Geometry check sheet. Reference: the model listing, model coordinates, mm. A direction names the side the tool comes from. Round coordinates to 2 decimals unless told otherwise and drop trailing zeros. Write each loop counter-clockwise with the first axis right and the second up, starting at its lowest first coordinate (ties: lowest second). Pieces come first, ordered by that corner, then holes.
Item 1: Cross-section at A-A (z = -9). Enter the section's corners in (x, y) (3 decimals), then the cut area to 3 significant figures.
Item 2: Scan lines: probe 1 along X at (y, z) = (0, -8.5); probe 2 along Y at (x, z) = (-0.5, -11.25); probe 3 along Y at (x, z) = (1, -2.75). Record each from-to range of solid material in increasing order.
Item 3: Draft check along X on faces 3 (the face through (-3.3, -5.6, -3.2)), 4 (the face through (0, 0, -13)), 5 (the face through (3.32, 0.74, -5.6)), 6 (the face through (3.3, 5.6, -3.2)). Enter one of: pulls with the +X half, pulls with the -X half, needs draft (parallel to the pull), parting line crosses it, or undercut.
Item 4: Access from +Z, -Z, +X, -X, +Y, -Y to the whole of each face (thin tool, end or side, straight path). Record for faces 1 (the face through (1.3, -4.1, 0)), 2 (the face through (1.88, 5.96, -7.61)).
Item 5: Depth check by flat-ended pin: P1, Ø4, axis at x = 0, y = 0, coming from the +Z side; P2, Ø1.5, axis at x = -4.5, y = 2.5, coming from the -Z side; P3, Ø1.5, axis at x = -4, y = -3, coming from the +Z side; P4, Ø8, axis at y = -4, z = -10.5, coming from the +X side. Enter the tip coordinate at first touch or a pass-through.
Item 6: Cross-section at B-B (z = -14). Enter the section's corners in (x, y), then the cut area to 3 significant figures.
from build123d import *

# Parameters (mm, degrees)
BOSS_EXTRUDE1_DEPTH = 15


with BuildPart() as part:
    # Sketch1 → Boss-Extrude1 (new body)
    with BuildSketch(Plane.XY):
        Polygon((0, 7.505553499), (-6.5, 3.75277675), (-6.5, -3.75277675), (0, -7.505553499), (6.5, -3.75277675), (6.5, 3.75277675), align=None)
    extrude(amount=-BOSS_EXTRUDE1_DEPTH)

    # Sketch2 → Cut-Revolve7 (revolve, cut)
    with BuildSketch(Plane(origin=(0, 0, 0), x_dir=(0, 0, -1), z_dir=(1, 0, 0))):
        with BuildLine():
            Line((16, 0), (15, 0))
            ThreePointArc((15, 0), (13.169417382, 4.419417382), (8.75, 6.25))
            Line((8.75, 6.25), (6.5, 6.25))
            Line((6.5, 6.25), (6.5, 30.553605498))
            Line((6.5, 30.553605498), (16, 30.553605498))
            Line((16, 30.553605498), (16, 0))
        make_face()
    revolve(axis=Axis((0, 0, 0), (0, 0, -1)), mode=Mode.SUBTRACT)

    # Sketch3 → Cut-Revolve8 (revolve, cut)
    with BuildSketch(Plane(origin=(0, 0, 0), x_dir=(0, 0, -1), z_dir=(1, 0, 0)), mode=Mode.PRIVATE) as cut_revolve8_sk:
        Polygon((5.775105849, 7.505553499), (6.5, 7.505553499), (6.5, 6.25), align=None)
        Polygon((0, 6.25), (0, 7.505553499), (0.724894151, 7.505553499), align=None)
    revolve(cut_revolve8_sk.sketch.rotate(Axis((0, 0, 0), (0, 0, -1)), 90), axis=Axis((0, 0, 0), (0, 0, -1)), mode=Mode.SUBTRACT)

    # Sketch4 → Cut-Revolve9 (revolve, cut)
    with BuildSketch(Plane(origin=(0, 0, 0), x_dir=(0, 0, -1), z_dir=(1, 0, 0)), mode=Mode.PRIVATE) as cut_revolve9_sk:
        Polygon((0, 4.1), (0.404145188, 3.4), (10.65, 3.4), (13, 0), (0, 0), align=None)
    revolve(cut_revolve9_sk.sketch.rotate(Axis((0, 0, 0), (0, 0, -1)), 180), axis=Axis((0, 0, 0), (0, 0, -1)), mode=Mode.SUBTRACT)


solid = part.part
Resolved:
1. outline: circle Ø12.49 at (0, 0); hole circle Ø6.8 at (0, 0)
1. area: 86.2 mm2
2. probe 1: x = -6.25 to -3.4, 3.4 to 6.25
2. probe 2: y = -5.71 to -2.48, 2.48 to 5.71
2. probe 3: y = -6.93 to -3.25, 3.25 to 6.93
3. face 3: pulls with the -X half
3. face 4: undercut
3. face 5: undercut
3. face 6: pulls with the +X half
4. face 1: +Z, +X, -X, +Y, -Y
4. face 2: -Z
5. P1: stops at z = -11.62
5. P2: stops at z = -13.19
5. P3: stops at z = 0
5. P4: stops at x = 6.24
6. outline: circle Ø6.78 at (0, 0)
6. area: 36.1 mm2
